```python
from build123d import *

# Parameters (mm, degrees)
F0_R     = 31.75
F1_DEPTH = 64
F2_R     = 19.7125485486
F3_DEPTH = 30
F5_DEPTH = 30
F6_R     = 5.5
F7_DEPTH = 35
F8_R     = 5.5
F9_DEPTH = 35


# Not quite as in the source:
# - the program builds the solid bodies; features that only make, move or delete a surface that nothing else refers to are left out


with BuildPart() as f1:
    # F0 (on Front) → F1 (new body)
    with BuildSketch(Plane.XZ):
        Circle(F0_R)
    extrude(amount=F1_DEPTH)

    # F2 (on face) → F3 (cut)
    with BuildSketch(Plane.XZ.offset(64)):
        Circle(F2_R)
    extrude(amount=-F3_DEPTH, mode=Mode.SUBTRACT)

    # F4 (on face) → F5 (cut)
    with BuildSketch(Plane(origin=(0, 0, 0), x_dir=(-1, 0, 0), z_dir=(0, 1, 0))):
        with BuildLine():
            Line((-30.8514586365, -7.5), (30.8514586365, -7.5))
            ThreePointArc((30.8514586365, -7.5), (31.5245643246, -3.7768166682), (31.75, 0))
            ThreePointArc((31.75, 0), (31.5245643246, 3.7768166682), (30.8514586365, 7.5))
            Line((30.8514586365, 7.5), (-30.8514586365, 7.5))
            ThreePointArc((-30.8514586365, 7.5), (-31.75, 0), (-30.8514586365, -7.5))
        make_face()
    extrude(amount=-F5_DEPTH, mode=Mode.SUBTRACT)

    # F6 (on Top) → F7 (cut, symmetric)
    with BuildSketch(Plane.XY):
        with Locations((0, -49)):
            Circle(F6_R)
    extrude(amount=F7_DEPTH, both=True, mode=Mode.SUBTRACT)

    # F8 (on Top) → F9 (cut, symmetric)
    with BuildSketch(Plane.XY):
        with Locations((0, -15)):
            Circle(F8_R)
    extrude(amount=F9_DEPTH, both=True, mode=Mode.SUBTRACT)


solid = f1.part
```
Model file for the job. Use its own axes, mm. A direction names the side the tool comes from. Round coordinates to 2 decimals unless told otherwise and drop trailing zeros. Write each loop counter-clockwise with the first axis right and the second up, starting at its lowest first coordinate (ties: lowest second). Pieces come first, ordered by that corner, then holes. Notation, with made-up numbers: (-15.75, 78) - (39.25, 78) arc R33 ccw to (39.25, 114) - close; hole circle Ø6 at (28, -29.5). An arc over 180 degrees is marked (long way). One line per item, written item: value.
(1) Cut at A-A, the plane y = -49. Give the cut face in (x, z).
Values follow:
outline: (-5.5, -31.27) - (-5.5, -18.93) arc R19.71 cw to (-5.5, 18.93) - (-5.5, 31.27) arc R31.75 ccw to start; (5.5, -31.27) arc R31.75 ccw to (5.5, 31.27) - (5.5, 18.93) arc R19.71 cw to (5.5, -18.93) - close
(2) Cut at D-D, the plane z = 0. Give the cut face in (x, y), plus the area to 3 significant figures.
Values follow:
outline: (-31.75, -64) - (-19.71, -64) - (-19.71, -34) - (19.71, -34) - (19.71, -64) - (31.75, -64) - (31.75, -30) - (-31.75, -30) - close
area: 976 mm²
(3) Drop flat-ended pins along their axis: P1, Ø15, axis at x = -14.5, y = -15.5, coming from the +Z side; P2, Ø5, axis at x = -16, y = -20, coming from the -Z side; P3, Ø2, axis at y = -54.5, z = -18.5, coming from the +X side; P4, Ø9, axis at x = -0.5, y = -15, coming from the -Z side. Give the stop position or say it passes through.
Values follow:
P1: stops at z = 30.97
P2: stops at z = -28.74
P3: stops at x = 26.49
P4: passes through
(4) 3-axis set-ups, long thin cutter, end or side, ignore diameter. For faces 1 (the cylindrical face through (-1.19, -20.37, -19.46)), 2 (the cylindrical face through (9.096, -49.21, -17.488)), 3 (the flat face through (0, -8, 7.5)): which of +Z, -Z, +X, -X, +Y, -Y reach the whole face in a straight line?
Values follow:
face 1: +Z, -Z
face 2: -Y
face 3: +X, -X, +Y
(5) Two-plate mould, pull along Z, no slides. Class faces 4 (the cylindrical face through (29.33, -31.55, -12.16)), 5 (the flat face through (0, -30, 0)), 6 (the flat face through (0, 0, -17)), 7 (the flat face through (0, -34, 0)): pulls with the +Z half, pulls with the -Z half, needs draft (parallel to the pull), parting line crosses it, or undercut.
Values follow:
face 4: parting line crosses it
face 5: undercut
face 6: needs draft
face 7: undercut
(6) Wall check: probe 1 along Y at (x, z) = (0, 21); probe 2 along Y at (x, z) = (0, 12.75); probe 3 along X at (y, z) = (-18, 17). Give the ranges that are in metal, low to high.
Values follow:
probe 1: y = -64 to -54.5, -43.5 to -20.5, -9.5 to 0
probe 2: y = -34 to -20.5, -9.5 to 0
probe 3: x = -26.82 to -4.61, 4.61 to 26.82
(7) Cut at B-B, the plane x = 0. Give the cut face in (y, z).
Values follow:
outline: (-64, -31.75) - (-54.5, -31.75) - (-54.5, -19.71) - (-64, -19.71) - close; (-64, 19.71) - (-54.5, 19.71) - (-54.5, 31.75) - (-64, 31.75) - close; (-43.5, -31.75) - (-20.5, -31.75) - (-20.5, -7.5) - (-30, -7.5) - (-30, 7.5) - (-20.5, 7.5) - (-20.5, 31.75) - (-43.5, 31.75) - (-43.5, 19.71) - (-34, 19.71) - (-34, -19.71) - (-43.5, -19.71) - close; (-9.5, -31.75) - (0, -31.75) - (0, -7.5) - (-9.5, -7.5) - close; (-9.5, 7.5) - (0, 7.5) - (0, 31.75) - (-9.5, 31.75) - close
(8) Cut at C-C, the plane y = -15. Give the cut face in (x, z), plus the area to 3 significant figures.
Values follow:
outline: (-30.85, -7.5) arc R31.75 ccw to (-5.5, -31.27) - (-5.5, -7.5) - close; (-30.85, 7.5) - (-5.5, 7.5) - (-5.5, 31.27) arc R31.75 ccw to start; (5.5, -31.27) arc R31.75 ccw to (30.85, -7.5) - (5.5, -7.5) - close; (5.5, 7.5) - (30.85, 7.5) arc R31.75 ccw to (5.5, 31.27) - close
area: 1,690 mm²
